Design review of the part built by this model. Coordinates are the model's own, in mm. A direction names the side the tool comes from. Coordinates: 2 decimals unless noted, no trailing zeros. Write each loop counter-clockwise with the first axis right and the second up, starting at its lowest first coordinate (ties: lowest second). Pieces come first, ordered by that corner, then holes. Notation, with made-up numbers: (-16, 59) -> (43, 59) arc R10 cw to (43, 72) -> close; hole circle Ø7 at (61.5, 33.25). An arc over 180 degrees is marked (long way). Write item = value, one per line. Start each with the question number.
```python
from build123d import *

# Parameters (mm, degrees)
F0_W     = 118
F0_H     = 30
F1_DEPTH = 35
F2_W     = 14
F2_H     = 14
F3_DEPTH = 33
F3_TAPER = 1
F4_W     = 110
F4_H     = 27
F5_DEPTH = 30


with BuildPart() as f1:
    # F0 (on Top) → F1 (new body)
    with BuildSketch(Plane.XY):
        with Locations((-5.2966810763, -25.8255312847)):
            Rectangle(F0_W, F0_H)
    extrude(amount=F1_DEPTH)

    # F2 (on face) → F3 (cut)
    with BuildSketch(Plane.XY.offset(35)):
        with Locations((-52.9612515788, -25.8255312847)):
            Rectangle(F2_W, F2_H)
        with Locations((-33.9612515788, -25.8255312847)):
            Rectangle(F2_W, F2_H)
        with Locations((-14.9612515788, -25.8255312847)):
            Rectangle(F2_W, F2_H)
        with Locations((4.0387484212, -25.8255312847)):
            Rectangle(F2_W, F2_H)
        with Locations((23.0387484212, -25.8255312847)):
            Rectangle(F2_W, F2_H)
        with Locations((42.0387484212, -25.8255312847)):
            Rectangle(F2_W, F2_H)
    extrude(amount=-F3_DEPTH, taper=F3_TAPER, mode=Mode.SUBTRACT)

    # F4 (on face) → F5 (cut)
    with BuildSketch(Plane.XZ.offset(40.8255312847)):
        with Locations((-5.2966810763, 17.5)):
            Rectangle(F4_W, F4_H)
    extrude(amount=-F5_DEPTH, mode=Mode.SUBTRACT)


solid = f1.part
```
(1) Mouldability with a two-part tool opening along Y and no side actions: class faces 4 (the face through (4, -26, 2)), 5 (the face through (49.703, -26, 17)), 6 (the face through (42, -26, 2)), 7 (the face through (-10, -40.826, 32)) as pulls with the +Y half, pulls with the -Y half, needs draft (parallel to the pull), parting line crosses it, or undercut.
(2) Take a section at A-A, the plane z = 9.5. State the section outline as (x, y) points, then the cut area to 3 significant figures.
(3) For pin 1 Ø4 at (x, y) = (-11.5, -27.5) entering from -Z; pin 2 Ø4 at (x, y) = (-34.5, -25.5) entering from +Z, all flat-tipped, find the tip position at first contact; note any pin that passes through.
(4) For faces 1 (the face through (-10, -10.826, 32)), 2 (the face through (-15, -26, 2)), 3 (the face through (-60.297, -26, 17)), list the 3-axis set-ups (+Z, -Z, +X, -X, +Y, -Y) from which the entire face can be reached by the end or side of a thin tool; tool diameter is ignored.
(5) Take a section at C-C, the plane x = -39. Count the separate pieces of the cut face and the enclosed holes in it, then the cut area to 3 significant figures.
(6) Take a section at B-B, the plane y = -35. State the section outline as (x, z) points, then the cut area to 3 significant figures.
(7) For line 1 (Z direction, x = -51.5, y = -18.5); line 2 (Y direction, x = -52, z = 32); line 3 (X direction, y = -38, z = 6.5), list the stretches that pass through material, from the lowest coordinate up.
Report:
q1.face_4 = undercut
q1.face_5 = needs draft
q1.face_6 = undercut
q1.face_7 = pulls with the -Y half
q2.outline = (-64.3, -40.83) -> (-60.3, -40.83) -> (-60.3, -10.83) -> (-64.3, -10.83) -> close; (49.7, -40.83) -> (53.7, -40.83) -> (53.7, -10.83) -> (49.7, -10.83) -> close
q2.area = 240 mm2
q3.pin_1 = 0
q3.pin_2 = 2
q4.face_1 = +Z, -Z, +X, -X, +Y
q4.face_2 = +Z
q4.face_3 = +Y, -Y
q5.separate_pieces = 3
q5.enclosed_holes = 0
q5.area = 159 mm2
q6.outline = (-64.3, 0) -> (53.7, 0) -> (53.7, 35) -> (-64.3, 35) -> close; hole (-60.3, 4) -> (49.7, 4) -> (49.7, 31) -> (-60.3, 31) -> close
q6.area = 1,160 mm2
q7.line_1 = 0 to 4, 31 to 35
q7.line_2 = -40.83 to -32.77, -18.88 to -10.83
q7.line_3 = -64.3 to -60.3, 49.7 to 53.7
